Read the model definition and answer for the solid it produces. Units are mm, in the model's axes. Face numbers are marked on the shaded views. Coordinates: 2 decimals unless noted, no trailing zeros. Loops run counter-clockwise (first coordinate to the right, second up) from the corner with the lowest first, then second, coordinate; pieces in that order, holes last. Notation, with made-up numbers: (23.25, -32.75) -> (35.25, -32.75) arc R25 ccw to (35.25, 1.25) -> close; hole circle Ø8 at (68.5, -9.75). An arc over 180 degrees is marked (long way). Answer as a JSON object with one key per item and string values. Group by question number.
Q1. Each of these flat-tipped pins is pushed along its axis until it touches: P1, Ø2, axis at x = -1, z = 23.5, coming from the +Y side; P2, Ø5, axis at x = -1.5, z = 4, coming from the +Y side; P3, Ø6.5, axis at x = -1.5, z = 25, coming from the +Y side; P4, Ø3, axis at x = 0, z = 25, coming from the +Y side. Where does it stop, or does it pass through?
Q2. Straight lines are drawn through the part: line 1 along Z through (x, y) = (0, -2.8); line 2 along Z through (x, y) = (0, -6.05); line 3 along X through (y, z) = (7, 7). For each, find the intervals that lie inside material, in ascending order. Write a range as [from, to].
Q3. The part is cut by section D-D on y = -5.5. Write down the section's boundary in (x, z), and give its area (3 significant figures).
Q4. The part is cut by section A-A on x = 0. Write down the section's boundary in (y, z), and give its area (3 significant figures).
Q5. The part is cut by section C-C on z = 5. Write down the section's boundary in (x, y).
Q6. Determine the mould class of the marked faces 1, 2, 3 and 4 for opening direction Z: released by +Z, released by -Z, zero draft, split by the parting line, or undercut.
Q7. The part is cut by section B-B on y = 6.25. Write down the section's boundary in (x, z), and give its area (3 significant figures).
from build123d import *

# Parameters (mm, degrees)
BOSS_EXTRUDE1_DEPTH = 30
FILLET1_R           = 0.8
SKETCH3_R           = 3
CUT_EXTRUDE1_DEPTH  = 12.5
SKETCH4_R           = 1.55
CUT_EXTRUDE2_DEPTH  = 35.882839707


with BuildPart() as part:
    # Sketch1 → Boss-Extrude1 (new body)
    with BuildSketch(Plane.XY):
        with BuildLine():
            Line((-5.25, 7.75), (-8.75, 7.75))
            Line((-8.75, 7.75), (-8.75, -7.75))
            Line((-8.75, -7.75), (8.75, -7.75))
            Line((8.75, -7.75), (8.75, 7.75))
            Line((8.75, 7.75), (5.25, 7.75))
            ThreePointArc((5.25, 7.75), (0, -1.306659276), (-5.25, 7.75))
        make_face()
    extrude(amount=BOSS_EXTRUDE1_DEPTH)

    # Fillet1
    fillet1_edges = [part.edges().sort_by_distance(p)[0] for p in [
        (-5.25, 7.75, 15),
        (5.25, 7.75, 15),
    ]]
    fillet(fillet1_edges, radius=FILLET1_R)

    # Sketch3 → Cut-Extrude1 (cut)
    with BuildSketch(Plane(origin=(0, 7.75, 0), x_dir=(1, 0, 0), z_dir=(0, 1, 0))):
        with Locations(Location((0, -5, 0), (0, 0, 180))):
            Circle(SKETCH3_R)
        with Locations(Location((0, -25, 0), (0, 0, 180))):
            Circle(SKETCH3_R)
    extrude(amount=-CUT_EXTRUDE1_DEPTH, mode=Mode.SUBTRACT)

    # Sketch4 → Cut-Extrude2 (cut, through all)
    with BuildSketch(Plane(origin=(0, 7.75, 0), x_dir=(1, 0, 0), z_dir=(0, 1, 0))):
        with Locations(Location((0, -5, 0), (0, 0, 180))):
            Circle(SKETCH4_R)
        with Locations(Location((0, -25, 0), (0, 0, 180))):
            Circle(SKETCH4_R)
    extrude(amount=-CUT_EXTRUDE2_DEPTH, mode=Mode.SUBTRACT)


solid = part.part
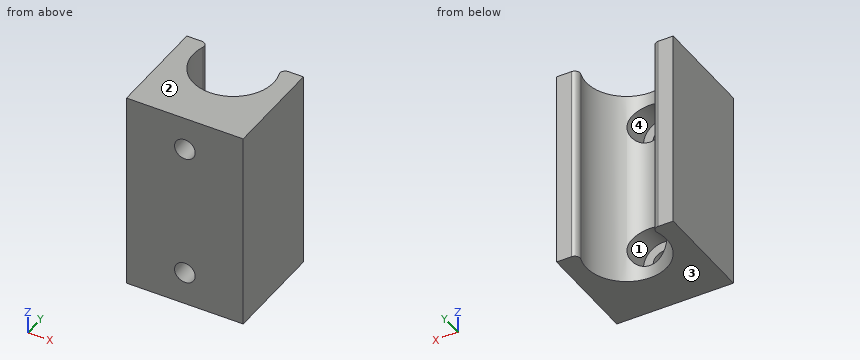
Final values:
{
 "1": {"P1": "stops at y = -4.75", "P2": "stops at y = 0.2", "P3": "stops at y = 1", "P4": "passes through"},
 "2": {"line 1": "z = [0, 2], [8, 22], [28, 30]", "line 2": "z = [0, 3.45], [6.55, 23.45], [26.55, 30]", "line 3": "x = [-8.75, -5.69], [5.69, 8.75]"},
 "3": {"outline": "(-8.75, 0) -> (8.75, 0) -> (8.75, 30) -> (-8.75, 30) -> close; hole circle Ø3.1 at (0, 5); hole circle Ø3.1 at (0, 25)", "area": "510 mm2"},
 "4": {"outline": "(-7.75, 0) -> (-1.31, 0) -> (-1.31, 2) -> (-4.75, 2) -> (-4.75, 3.45) -> (-7.75, 3.45) -> close; (-7.75, 6.55) -> (-4.75, 6.55) -> (-4.75, 8) -> (-1.31, 8) -> (-1.31, 22) -> (-4.75, 22) -> (-4.75, 23.45) -> (-7.75, 23.45) -> close; (-7.75, 26.55) -> (-4.75, 26.55) -> (-4.75, 28) -> (-1.31, 28) -> (-1.31, 30) -> (-7.75, 30) -> close", "area": "133 mm2"},
 "5": {"outline": "(-8.75, -7.75) -> (-1.55, -7.75) -> (-1.55, -4.75) -> (-3, -4.75) -> (-3, -0.51) arc R6.05 cw to (-5.73, 6.69) arc R0.8 ccw to (-6.48, 7.75) -> (-8.75, 7.75) -> close; (1.55, -7.75) -> (8.75, -7.75) -> (8.75, 7.75) -> (6.48, 7.75) arc R0.8 ccw to (5.73, 6.69) arc R6.05 cw to (3, -0.51) -> (3, -4.75) -> (1.55, -4.75) -> close"},
 "6": {"face 1": "undercut", "face 2": "released by +Z", "face 3": "released by -Z", "face 4": "undercut"},
 "7": {"outline": "(-8.75, 0) -> (-5.86, 0) -> (-5.86, 30) -> (-8.75, 30) -> close; (5.86, 0) -> (8.75, 0) -> (8.75, 30) -> (5.86, 30) -> close", "area": "173 mm2"}
}
